Here's how the part is built. I have some questions about the finished solid (model axes, mm). Face numbers are marked on the shaded views. Round coordinates to 2 decimals unless told otherwise and drop trailing zeros. Write each loop counter-clockwise with the first axis right and the second up, starting at its lowest first coordinate (ties: lowest second). Pieces come first, ordered by that corner, then holes. Notation, with made-up numbers: (9, 45) - (44, 45) arc R20 cw to (44, 70) - close; hole circle Ø6 at (-6.75, 3). An arc over 180 degrees is marked (long way). One line per item, written item: value. Start each with the question number.
Item 1: Imagine slicing it at D-D, the plane y = 0. Please give me the cut outline in (x, z) (3 decimals), then the cut area to 3 significant figures.
Item 2: Imagine slicing it at B-B, the plane z = 1.95. Please give me the cut outline in (x, y), then the cut area to 3 significant figures.
Item 3: Imagine slicing it at C-C, the plane x = 1. Please give me the cut outline in (y, z) (3 decimals), then the cut area to 3 significant figures.
Item 4: If I drill on line 1 (Y direction, x = 0, z = 3.2); line 2 (X direction, y = -4, z = 0.85); line 3 (Y direction, x = 38.5, z = 4.1), over which ranges is the centre line in solid material (lowest first)?
Item 5: Thinking about a two-plate mould opening in X: for the marked faces 1, 2 and 3, which applies, released by +X, released by -X, zero draft, split by the parting line, or undercut?
Item 6: Imagine slicing it at A-A, the plane y = -2.5. Please give me the cut outline in (x, z) (3 decimals), then the cut area to 3 significant figures.
```python
from build123d import *

# Parameters (mm, degrees)
SKETCH1_R           = 1.7526
BOSS_EXTRUDE1_DEPTH = 4.445


with BuildPart() as part:
    # Sketch1 → Boss-Extrude1 (new body)
    with BuildSketch(Plane.XY):
        with BuildLine():
            Line((45.097053324, -5.527793834), (45.097053324, 2.092206166))
            ThreePointArc((45.097053324, 2.092206166), (21.378517637, 13.276466986), (-4.510590735, 9.103854745))
            ThreePointArc((-4.510590735, 9.103854745), (-8.328542576, -5.819018694), (6.997053324, -7.366603341))
            ThreePointArc((6.997053324, -7.366603341), (25.705466674, 0.630452091), (45.097053324, -5.527793834))
        make_face()
        Circle(SKETCH1_R, mode=Mode.SUBTRACT)
    extrude(amount=BOSS_EXTRUDE1_DEPTH)


solid = part.part
```
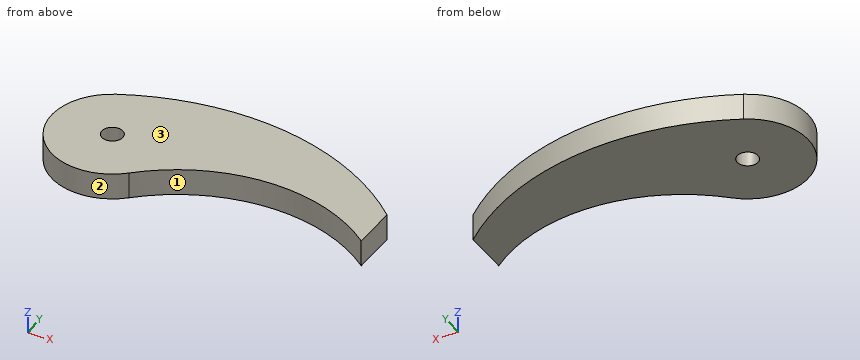
Values follow:
1. outline: (-10.16, 0) - (-1.753, 0) - (-1.753, 4.445) - (-10.16, 4.445) - close; (1.753, 0) - (20.919, 0) - (20.919, 4.445) - (1.753, 4.445) - close; (33.308, 0) - (45.097, 0) - (45.097, 4.445) - (33.308, 4.445) - close
1. area: 175 mm^2
2. outline: (-4.51, 9.1) arc R10.16 ccw (long way) to (7, -7.37) arc R29.21 cw to (45.1, -5.53) - (45.1, 2.09) arc R44.34 ccw to start; hole circle Ø3.51 at (0, 0)
2. area: 775 mm^2
3. outline: (-10.111, 0) - (-1.439, 0) - (-1.439, 4.445) - (-10.111, 4.445) - close; (1.439, 0) - (11.386, 0) - (11.386, 4.445) - (1.439, 4.445) - close
3. area: 82.8 mm^2
4. line 1: y = -10.16 to -1.75, 1.75 to 11.04
4. line 2: x = -9.34 to 11.28, 42.95 to 45.1
4. line 3: y = -1.65 to 7.08
5. face 1: undercut
5. face 2: split by the parting line
5. face 3: zero draft
6. outline: (-9.848, 0) - (13.89, 0) - (13.89, 4.445) - (-9.848, 4.445) - close; (40.337, 0) - (45.097, 0) - (45.097, 4.445) - (40.337, 4.445) - close
6. area: 127 mm^2
